```python
from build123d import *

# Parameters (mm, degrees)
F0_W      = 90
F0_H      = 130
F0_W_2    = 45
F0_H_2    = 110
F1_DEPTH  = 23
F2_W      = 3.5
F2_H      = 130
F2_W_2    = 23
F3_DEPTH  = 10
F5_DEPTH  = 4
F6_W      = 5.5
F6_H      = 10
F6_W_2    = 3.1640307605
F6_W_3    = 2.3359692395
F6_W_4    = 10
F6_W_5    = 20
F6_H_2    = 40.1
F6_R      = 3
F7_DEPTH  = 15.5
F9_D      = 3.3
F9_DEPTH  = 40
F9_TIP    = 0.9914200214
F10_D     = 3.3
F10_DEPTH = 40
F10_TIP   = 0.9914200214
F12_D     = 3.3
F12_DEPTH = 40
F12_TIP   = 0.9914200214
F14_D     = 4.4
F14_DEPTH = 10
F14_TIP   = 1.3218933619
F15_R     = 2.2
F16_DEPTH = 4


with BuildPart() as f1:
    # F0 (on Front) → F1 (new body)
    with BuildSketch(Plane.XZ):
        with Locations((10.2966074646, 21.924110651)):
            Rectangle(F0_W, F0_H)
        with Locations((2.7966074646, 21.924110651)):
            Rectangle(F0_W_2, F0_H_2, mode=Mode.SUBTRACT)
    extrude(amount=F1_DEPTH)

    # F2 (on face) → F3 (join)
    with BuildSketch(Plane(origin=(-34.7033925354, 0, 0), x_dir=(0, -1, 0), z_dir=(-1, 0, 0))):
        with Locations((-1.75, 21.924110651)):
            Rectangle(F2_W, F2_H)
        with Locations((11.5, 21.924110651)):
            Rectangle(F2_W_2, F2_H)
        with Locations((24.75, 21.924110651)):
            Rectangle(F2_W, F2_H)
    extrude(amount=F3_DEPTH)

    # F4 (on face) → F5 (cut)
    with BuildSketch(Plane.XZ.offset(23)):
        Polygon((55.2966074646, -43.075889349), (55.2966074646, 86.924110651), (25.2966074646, 86.924110651), (25.2966074646, 76.924110651), (25.2966074646, -33.075889349), (25.2966074646, -43.075889349), align=None)
    extrude(amount=-F5_DEPTH, mode=Mode.SUBTRACT)

    # F6 (on face) → F7 (cut)
    with BuildSketch(Plane.XZ.offset(19)):
        Polygon((42.132576704, 65.924110651), (27.632576704, 65.924110651), (27.632576704, 56.424110651), (33.132576704, 56.424110651), (33.132576704, 46.424110651), (27.632576704, 46.424110651), (27.632576704, 36.924110651), (42.132576704, 36.924110651), (52.132576704, 36.924110651), (52.132576704, 65.924110651), align=None)
        with Locations((30.382576704, 51.424110651)):
            Rectangle(F6_W, F6_H)
        with Locations((23.7145920843, 51.424110651)):
            Rectangle(F6_W_2, F6_H)
        with Locations((26.4645920843, 51.424110651)):
            Rectangle(F6_W_3, F6_H)
        with Locations((47.132576704, 70.924110651)):
            Rectangle(F6_W_4, F6_H)
        with Locations((47.132576704, 31.924110651)):
            Rectangle(F6_W_4, F6_H)
        with Locations((35.2966074646, -5.2936900675)):
            Rectangle(F6_W_5, F6_H_2)
        with Locations((35.2966074646, -15.2936900675)):
            Circle(F6_R, mode=Mode.SUBTRACT)
        with Locations((35.2966074646, 4.7063099325)):
            Circle(F6_R, mode=Mode.SUBTRACT)
    extrude(amount=-F7_DEPTH, mode=Mode.SUBTRACT)

    # F9
    with Locations(Plane.XZ.offset(19)):
        with Locations((35.2966074646, 4.7063099325), (35.2966074646, -15.2936900675)):
            Hole(F9_D / 2, depth=F9_DEPTH)
            with Locations((0, 0, -(F9_DEPTH + F9_TIP / 2))):  # 118° drill point
                Cone(0, F9_D / 2, F9_TIP, mode=Mode.SUBTRACT)

    # F10
    with Locations(Plane(origin=(0, 0, 0), x_dir=(1, 0, 0), z_dir=(0, 1, 0))):
        with Locations((35.2966074646, -76.924110651)):
            Hole(F10_D / 2, depth=F10_DEPTH)
            with Locations((0, 0, -(F10_DEPTH + F10_TIP / 2))):  # 118° drill point
                Cone(0, F10_D / 2, F10_TIP, mode=Mode.SUBTRACT)

    # F12 (one way)
    with BuildSketch(Plane.YZ.offset(-19.7033925354)):
        with Locations((-11.5, 56.924110651), (-11.5, -13.075889349)):
            Circle(F12_D / 2)
    extrude(amount=-F12_DEPTH, mode=Mode.SUBTRACT)
    with Locations(Plane.YZ.offset(-19.7033925354)):
        with Locations((-11.5, 56.924110651), (-11.5, -13.075889349)):
            with Locations((0, 0, -(F12_DEPTH + F12_TIP / 2))):  # 118° drill point
                Cone(0, F12_D / 2, F12_TIP, mode=Mode.SUBTRACT)

    # F14
    with Locations(Plane(origin=(0, 0, -43.075889349), x_dir=(1, 0, 0), z_dir=(0, 0, -1))):
        with Locations((-14.7033925354, 11.5)):
            Hole(F14_D / 2, depth=F14_DEPTH)
            with Locations((0, 0, -(F14_DEPTH + F14_TIP / 2))):  # 118° drill point
                Cone(0, F14_D / 2, F14_TIP, mode=Mode.SUBTRACT)

    # F15 (on face) → F16 (cut)
    with BuildSketch(Plane.XY.offset(-33.075889349)):
        Polygon((-11.1772465223, -9.524560281), (-14.6511005092, -7.4585481157), (-18.1772465223, -9.4339878346), (-18.2295385486, -13.475439719), (-14.7556845617, -15.5414518843), (-11.2295385486, -13.5660121654), align=None)
        with Locations((-14.7033925354, -11.5)):
            Circle(F15_R, mode=Mode.SUBTRACT)
    extrude(amount=-F16_DEPTH, mode=Mode.SUBTRACT)


solid = f1.part
```
Here's how the part is built. I have some questions about the finished solid (model axes, mm). A direction names the side the tool comes from. Coordinates: 2 decimals unless noted, no trailing zeros. Loops run counter-clockwise (first coordinate to the right, second up) from the corner with the lowest first, then second, coordinate; pieces in that order, holes last. Notation, with made-up numbers: (-17.75, 0) - (-0.75, 0) arc R20 ccw to (-0.75, 33) - close; hole circle Ø10 at (17, 66.5). An arc over 180 degrees is marked (long way). Return JSON: item names as keys, results as strings. Group by question number.
Item 1: On a 3-axis mill with a long thin cutter (end or side, diameter ignored), from which of +Z, -Z, +X, -X, +Y, -Y can I reach the whole of each face in a straight line? I mean faces 1 (the face through (42.133, -11, 32)), 2 (the face through (-32.028, -9.976, -13.708)), 3 (the face through (-16.52, -14.49, -35.05)), 4 (the face through (-19.703, -11, 21)). Say none if no direction works.
Item 2: I need wall thicknesses on line 1 (X direction, y = -14, z = 45); line 2 (X direction, y = -8, z = 73); line 3 (Z direction, x = -38.5, y = -11.5). Which ranges of each line are inside material? Lowest first, please. Write a range as from..to.
Item 3: Will these pins go through, and if not, where does the flat tip stop? P1, Ø3, axis at y = -24, z = -3.5, coming from the +X side; P2, Ø6, axis at x = 37.5, z = -4, coming from the -Y side; P3, Ø4.5, axis at x = 35.3, z = -15.29, coming from the -Y side.
Item 4: If we section it at C-C on z = 49.5: Write out the boundary of the cut face in (x, y).
Item 5: If we section it at B-B on x = 12.5: Write out the boundary of the cut face in (y, z).
Item 6: If we section it at D-D on y = -21.25: Write out the boundary of the cut face in (x, z).
Item 7: If we section it at A-A on z = -20: Write out the boundary of the cut face in (x, y), and give its area (3 significant figures).
Item 8: We'd pull the mould along Y, two halves only. Please class faces 5 (the face through (37, -19, 3)), 6 (the face through (-12.506, -11.597, -40.034)), 7 (the face through (33.772, -9.367, 4.074)): +Y half, -Y half, draft (parallel to the pull), parting line (faces both ways), or undercut.
Calculated:
{
 "1": {"face 1": "-Y", "face 2": "-X", "face 3": "none", "face 4": "+Y, -Y"},
 "2": {"line 1": "x = -44.7..-19.7, 25.3..27.63, 52.13..55.3", "line 2": "x = -44.7..-19.7, 25.3..42.13, 52.13..55.3", "line 3": "z = -43.08..-14.73, -11.43..55.27, 58.57..86.92"},
 "3": {"P1": "stops at x = -19.7", "P2": "stops at y = -3.5", "P3": "stops at y = -19"},
 "4": {"outline": "(-44.7, -26.5) - (-34.7, -26.5) - (-34.7, -23) - (-19.7, -23) - (-19.7, 0) - (-34.7, 0) - (-34.7, 3.5) - (-44.7, 3.5) - close; (25.3, -3.5) - (52.13, -3.5) - (52.13, -19) - (55.3, -19) - (55.3, 0) - (25.3, 0) - close"},
 "5": {"outline": "(-23, -43.08) - (0, -43.08) - (0, -33.08) - (-23, -33.08) - close; (-23, 76.92) - (0, 76.92) - (0, 86.92) - (-23, 86.92) - close"},
 "6": {"outline": "(-44.7, -43.08) - (25.3, -43.08) - (25.3, -33.08) - (-19.7, -33.08) - (-19.7, 76.92) - (25.3, 76.92) - (25.3, 86.92) - (-44.7, 86.92) - close"},
 "7": {"outline": "(-44.7, -26.5) - (-34.7, -26.5) - (-34.7, -23) - (-19.7, -23) - (-19.7, 0) - (-34.7, 0) - (-34.7, 3.5) - (-44.7, 3.5) - close; (25.3, -3.5) - (45.3, -3.5) - (45.3, -19) - (55.3, -19) - (55.3, 0) - (25.3, 0) - close", "area": "905 mm^2"},
 "8": {"face 5": "-Y half", "face 6": "undercut", "face 7": "draft"}
}
